Geometry: final body of the model. Coordinates: model frame, mm. A direction names the side the tool comes from. Coordinates: 2 decimals unless noted, no trailing zeros. Loops run counter-clockwise (first coordinate to the right, second up) from the corner with the lowest first, then second, coordinate; pieces in that order, holes last. Notation, with made-up numbers: (26.5, 18) - (35.5, 18) arc R6 cw to (35.5, 23) - close; hole circle Ø1 at (-39.75, 72). An arc over 180 degrees is marked (long way). Put each result on its own line as item: value. Start each with the question number.
1) Reachability of faces 1 (the flat face through (14.461, -10, 18)), 2 (the flat face through (-14.461, -10, 18)), 3 (the flat face through (0, -42.857, 32)) from +Z, -Z, +X, -X, +Y, -Y: full face, straight path, thin tool, end or side. Return the list, or none.
2) Contact query for flat-ended pins moving along their axis: pin 1 Ø12 at (x, y) = (16, -31) entering from +Z; pin 2 Ø8.5 at (x, z) = (1.5, 29) entering from -Y; pin 3 Ø15 at (x, y) = (11.5, -30.5) entering from +Z; pin 4 Ø1.5 at (x, y) = (-14, 21) entering from -Z. Output: stop coordinate, or through.
3) Section D-D on z = 44.5. Output: boundary loops of the cut face in (x, y).
4) Section C-C on x = 3.5. Output: boundary loops of the cut face in (y, z), and give its area (3 significant figures).
5) Section B-B on y = -32.5. Output: boundary loops of the cut face in (x, z).
6) Material intervals for line 1 along Y through (x, z) = (0, 7.5); line 2 along Y through (x, z) = (-9.5, 42.5); line 3 along Z through (x, y) = (23.5, 27.5), sorted ascending. Write a range as from..to.
7) Section A-A on z = 37. Output: boundary loops of the cut face in (x, y), and give its area (3 significant figures).
8) Draft query along X for faces 4 (the flat face through (24.816, -1, 6)), 5 (the cylindrical face through (-1.106, -69.873, 6.261)), 6 (the flat face through (0, 42.857, 32)). Return one class per face: +X half, -X half, draft (parallel to the pull), parting line (faces both ways), or undercut.
```python
from build123d import *

# Parameters (mm, degrees)
F0_R          = 5.1422573348
F0_W          = 49.6318712831
F0_H          = 106.9652438164
F0_R_2        = 5.1025471004
F1_DEPTH      = 12.7
F2_W          = 28.9213098586
F2_H          = 85.7132077217
F3_DEPTH      = 50.8
F4_T1_DEPTH   = 161.9132077217
F5_R          = 7.0462908342
F6_DEPTH      = 101.6
F7_W          = 39.3632203341
F7_H          = 41.8217248726
F8_DEPTH      = 50.8
F8_DEPTH_BACK = 25.4


# Not quite as in the source:
# - a fillet or chamfer that OpenCascade refuses, or shapes differently, is made with other operations: its cross-section is extruded or revolved along the edge and cut away or added


with BuildPart() as f1:
    # F0 (on Top) → F1 (new body)
    with BuildSketch(Plane.XY):
        with BuildLine():
            ThreePointArc((24.8159356415, 53.4826219082), (0, 78.2985575497), (-24.8159356415, 53.4826219082))
            Line((-24.8159356415, 53.4826219082), (24.8159356415, 53.4826219082))
        make_face()
        with Locations((0, 64.6070018411)):
            Circle(F0_R, mode=Mode.SUBTRACT)
        Rectangle(F0_W, F0_H)
        with BuildLine():
            Line((24.8159356415, -53.4826219082), (-24.8159356415, -53.4826219082))
            ThreePointArc((-24.8159356415, -53.4826219082), (0, -78.2985575497), (24.8159356415, -53.4826219082))
        make_face()
        with Locations((0, -64.8922473192)):
            Circle(F0_R_2, mode=Mode.SUBTRACT)
    extrude(amount=F1_DEPTH)

    # F2 (on face) → F3 (join)
    with BuildSketch(Plane.XY.offset(12.7)):
        Rectangle(F2_W, F2_H)
    extrude(amount=F3_DEPTH)

    # F4: fillet of radius 15.24 on 2 edges, made by hand

    # F4_s2 → F4_t1 (cut)
    with BuildSketch(Plane.XZ.offset(-80.9566038609)):
        with BuildLine():
            ThreePointArc((14.4606549293, 48.26), (9.9969622746, 59.0363073453), (-0.7793450707, 63.5))
            Line((-0.7793450707, 63.5), (14.4606549293, 63.5))
            Line((14.4606549293, 63.5), (14.4606549293, 48.26))
        make_face()
        with BuildLine():
            ThreePointArc((-14.4606549293, 48.26), (-9.9969622746, 59.0363073453), (0.7793450707, 63.5))
            Line((0.7793450707, 63.5), (-14.4606549293, 63.5))
            Line((-14.4606549293, 63.5), (-14.4606549293, 48.26))
        make_face()
    extrude(amount=F4_T1_DEPTH, mode=Mode.SUBTRACT)

    # F5 (on face) → F6 (cut)
    with BuildSketch(Plane(origin=(0, 42.8566038609, 0), x_dir=(-1, 0, 0), z_dir=(0, 1, 0))):
        with Locations((0.7793450707, 48.26)):
            Circle(F5_R)
    extrude(amount=-F6_DEPTH, mode=Mode.SUBTRACT)

    # F7 (on face) → F8 (cut, two sides)
    with BuildSketch(Plane(origin=(-14.4606549293, 0, 0), x_dir=(0, -1, 0), z_dir=(-1, 0, 0))) as f8_sk:
        with Locations((0, 48.26)):
            Rectangle(F7_W, F7_H)
        with BuildLine():
            Line((19.681610167, 27.3491375637), (-19.681610167, 27.3491375637))
            ThreePointArc((-19.681610167, 27.3491375637), (0, 16.517771495), (19.681610167, 27.3491375637))
        make_face()
    extrude(amount=-F8_DEPTH, mode=Mode.SUBTRACT)
    extrude(f8_sk.sketch, amount=F8_DEPTH_BACK, mode=Mode.SUBTRACT)


solid = f1.part
```
Answer block:
1. face 1: +Z, +X, +Y, -Y
1. face 2: +Z, -X, +Y, -Y
1. face 3: +Z, +X, -X, -Y
2. pin 1: stops at z = 59.03
2. pin 2: stops at y = -42.86
2. pin 3: stops at z = 62.73
2. pin 4: stops at z = 0
3. outline: (-14.46, -42.86) - (-6.74, -42.86) - (-6.74, -19.68) - (-14.46, -19.68) - close; (-14.46, 19.68) - (-6.74, 19.68) - (-6.74, 42.86) - (-14.46, 42.86) - close; (5.18, -42.86) - (14.46, -42.86) - (14.46, -19.68) - (5.18, -19.68) - close; (5.18, 19.68) - (14.46, 19.68) - (14.46, 42.86) - (5.18, 42.86) - close
4. outline: (-78.05, 0) - (-68.61, 0) - (-68.61, 12.7) - (-78.05, 12.7) - close; (-61.18, 0) - (60.84, 0) - (60.84, 12.7) - (42.86, 12.7) - (42.86, 42.66) - (19.68, 42.66) - (19.68, 27.35) arc R23.3 cw to (-19.68, 27.35) - (-19.68, 42.66) - (-42.86, 42.66) - (-42.86, 12.7) - (-61.18, 12.7) - close; (-42.86, 53.86) - (-19.68, 53.86) - (-19.68, 62.89) - (-42.86, 62.89) - close; (19.68, 53.86) - (42.86, 53.86) - (42.86, 62.89) - (19.68, 62.89) - close; (68.37, 0) - (78.05, 0) - (78.05, 12.7) - (68.37, 12.7) - close
4. area: 3,880 mm²
5. outline: (-24.82, 0) - (24.82, 0) - (24.82, 12.7) - (14.46, 12.7) - (14.46, 48.26) arc R15.24 ccw to (0, 63.48) arc R15.24 ccw to (-14.46, 48.26) - (-14.46, 12.7) - (-24.82, 12.7) - close; hole circle Ø14.09 at (-0.78, 48.26)
6. line 1: y = -78.3..-69.99, -59.79..59.46, 69.75..78.3
6. line 2: y = -42.86..-19.68, 19.68..42.86
6. line 3: z = 0..12.7
7. outline: (-14.46, -42.86) - (14.46, -42.86) - (14.46, -19.68) - (-14.46, -19.68) - close; (-14.46, 19.68) - (14.46, 19.68) - (14.46, 42.86) - (-14.46, 42.86) - close
7. area: 1,340 mm²
8. face 4: +X half
8. face 5: undercut
8. face 6: draft
